Source: CAD feature listing. Evaluate the final solid. Frame: model axes, mm. A direction names the side the tool comes from. Give positions to 0.01 mm unless a question says otherwise; leave off trailing zeros. Loops run counter-clockwise (first coordinate to the right, second up) from the corner with the lowest first, then second, coordinate; pieces in that order, holes last.
from build123d import *

# Parameters (mm, degrees)
F1_DEPTH = 31.75
F2_R     = 10.16
F3_DEPTH = 166.371
F5_DEPTH = 166.371


with BuildPart() as f1:
    # F0 (on Front) → F1 (new body, symmetric)
    with BuildSketch(Plane.XZ):
        Polygon((-108.20795, 89.455473), (-108.20795, -75.371138), (58.16205, -75.371138), (58.16205, 92.395943), (39.11205, 92.395943), (39.11205, -37.714908), (-89.15795, -37.714908), (-89.15795, 89.455473), align=None)
        with BuildLine():
            Line((58.16205, -75.371138), (-108.20795, -75.371138))
            ThreePointArc((-108.20795, -75.371138), (-25.02295, -104.792049), (58.16205, -75.371138))
        make_face()
    extrude(amount=F1_DEPTH, both=True)

    # F2 (on face) → F3 (cut, through all)
    with BuildSketch(Plane(origin=(-108.20795, 0, 0), x_dir=(0, -1, 0), z_dir=(-1, 0, 0))):
        with Locations((0, 57.705473)):
            Circle(F2_R)
    extrude(amount=-F3_DEPTH, mode=Mode.SUBTRACT)

    # F4 (on face) → F5 (cut, through all)
    with BuildSketch(Plane.YZ.offset(58.16205)):
        with BuildLine():
            ThreePointArc((-31.75, 71.282387), (-0.077504, 85.238302), (31.75, 71.639605))
            Line((31.75, 71.639605), (31.75, 92.395943))
            Line((31.75, 92.395943), (-31.75, 92.395943))
            Line((-31.75, 92.395943), (-31.75, 71.282387))
        make_face()
    extrude(amount=-F5_DEPTH, mode=Mode.SUBTRACT)


solid = f1.part
1) Cut plane C-C (y = -23). Return loops of the section in (x, z).
Checks:
outline: (-108.21, -75.37) arc R132.31 ccw to (58.16, -75.37) - (58.16, 78.55) - (39.11, 78.55) - (39.11, -37.71) - (-89.16, -37.71) - (-89.16, 78.55) - (-108.21, 78.55) - close
2) Contact query for flat-ended pins moving along their axis: P1, Ø1.5, axis at x = -19, y = 11, coming from the +Z side; P2, Ø2, axis at y = 7, z = -77.5, coming from the -X side. Output: stop coordinate, or through.
Checks:
P1: stops at z = -37.71
P2: stops at x = -106.79
3) Pull-direction query (X, two-part tool) for faces 1 (the flat face through (-24, 0, -37.715)), 2 (the flat face through (-108.208, 0, 6)), 3 (the flat face through (-26, -31.75, -55)); classes: released by +X, released by -X, zero draft, split by the parting line, or undercut.
Checks:
face 1: undercut
face 2: released by -X
face 3: zero draft
4) Cut plane D-D (x = -40). Return loops of the section in (y, z).
Checks:
outline: (-31.75, -103.94) - (31.75, -103.94) - (31.75, -37.71) - (-31.75, -37.71) - close
5) Ray query, probe 1 along X at (y, z) = (-14.5, 33.5); probe 2 along Z at (x, y) = (47, 0); probe 3 along Z at (x, y) = (48.5, 0). Return the intervals inside material, ascending.
Checks:
probe 1: x = -108.21 to -89.16, 39.11 to 58.16
probe 2: z = -83.47 to 47.55, 67.87 to 85.24
probe 3: z = -82.48 to 47.55, 67.87 to 85.24
6) Cut plane A-A (z = 1). Return loops of the section in (x, y).
Checks:
outline: (-108.21, -31.75) - (-89.16, -31.75) - (-89.16, 31.75) - (-108.21, 31.75) - close; (39.11, -31.75) - (58.16, -31.75) - (58.16, 31.75) - (39.11, 31.75) - close
7) Cut plane B-B (y = -6). Return loops of the section in (x, z).
Checks:
outline: (-108.21, -75.37) arc R132.31 ccw to (58.16, -75.37) - (58.16, 49.51) - (39.11, 49.51) - (39.11, -37.71) - (-89.16, -37.71) - (-89.16, 49.51) - (-108.21, 49.51) - close; (-108.21, 65.9) - (-89.16, 65.9) - (-89.16, 84.8) - (-108.21, 84.8) - close; (39.11, 65.9) - (58.16, 65.9) - (58.16, 84.8) - (39.11, 84.8) - close
8) Reachability of faces 4 (the flat face through (39.112, 0, 25)), 5 (the flat face through (58.162, 0, 4)) from +Z, -Z, +X, -X, +Y, -Y: full face, straight path, thin tool, end or side. Return the list, or none.
Checks:
face 4: +Z, +Y, -Y
face 5: +Z, -Z, +X, +Y, -Y
